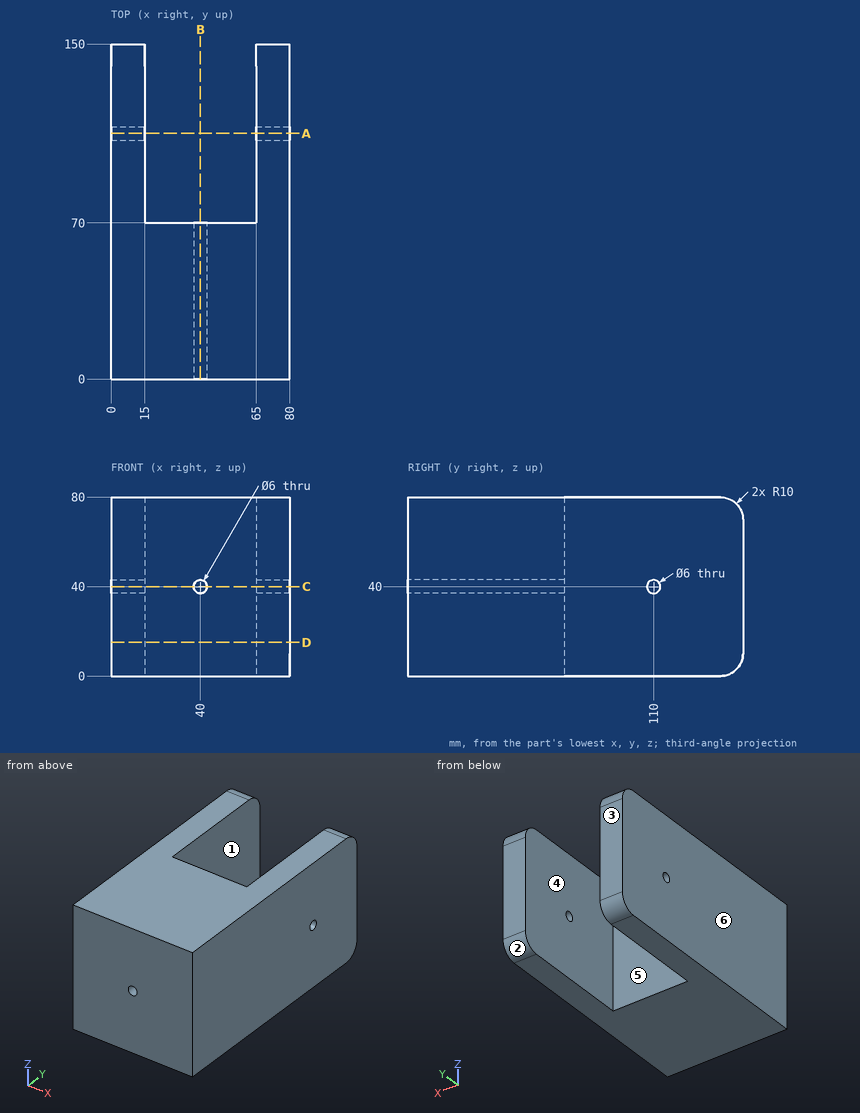
Geometry check sheet. Reference: drawing and pictorial views, mm from the part's lowest x, y, z. A direction names the side the tool comes from. Round coordinates to 2 decimals unless told otherwise and drop trailing zeros. Order: outer loops, then holes, each group sorted by start corner. A loop starts at its lowest first (then second) coordinate and runs counter-clockwise, first axis right, second up.
Q1. Cross-section at A-A, the plane y = 110. Enter the section's corners in (x, z).
Filled sheet:
outline: (0, 0) - (15, 0) - (15, 37) - (0, 37) - close; (0, 43) - (15, 43) - (15, 80) - (0, 80) - close; (65, 0) - (80, 0) - (80, 37) - (65, 37) - close; (65, 43) - (80, 43) - (80, 80) - (65, 80) - close
Q2. Draft check along X on the marked faces 3, 4, 5 and 6. Enter one of: pulls with the +X half, pulls with the -X half, needs draft (parallel to the pull), parting line crosses it, or undercut.
Filled sheet:
face 3: needs draft
face 4: undercut
face 5: undercut
face 6: pulls with the -X half
Q3. Set-up check for the marked faces 1 and 2: record each of +Z, -Z, +X, -X, +Y, -Y from which the full face is reachable in a straight line by a thin tool's end or side.
Filled sheet:
face 1: +Z, -Z, +Y
face 2: -Z, +X, -X, +Y
Q4. Cross-section at B-B, the plane x = 40. Enter the section's corners in (y, z).
Filled sheet:
outline: (0, 0) - (70, 0) - (70, 37) - (0, 37) - close; (0, 43) - (70, 43) - (70, 80) - (0, 80) - close
Q5. Scan lines: L1, parallel to Z at x = 40, y = 31; L2, parallel to Y at x = 77, z = 40; L3, parallel to X at y = 114, z = 60. Record each from-to range of solid material in increasing order.
Filled sheet:
L1: z = 0 to 37, 43 to 80
L2: y = 0 to 107, 113 to 150
L3: x = 0 to 15, 65 to 80
Q6. Cross-section at D-D, the plane z = 15. Enter the section's corners in (x, y).
Filled sheet:
outline: (0, 0) - (80, 0) - (80, 150) - (65, 150) - (65, 70) - (15, 70) - (15, 150) - (0, 150) - close
Q7. Cross-section at C-C, the plane z = 40. Enter the section's corners in (x, y).
Filled sheet:
outline: (0, 0) - (37, 0) - (37, 70) - (15, 70) - (15, 107) - (0, 107) - close; (0, 113) - (15, 113) - (15, 150) - (0, 150) - close; (43, 0) - (80, 0) - (80, 107) - (65, 107) - (65, 70) - (43, 70) - close; (65, 113) - (80, 113) - (80, 150) - (65, 150) - close
